from build123d import *

# Parameters (mm, degrees)
SKETCH_1_W      = 60
SKETCH_1_H      = 44
EXTRUDE_3_DEPTH = 2.5
SKETCH_4_R      = 1.5
EXTRUDE_4_DEPTH = 17.5
EXTRUDE_START   = -17.5
SKETCH_5_R      = 1.5
EXTRUDE_5_DEPTH = 17.5


with BuildPart() as part:
    # 草图1 → 凸台-拉伸3 (new body)
    with BuildSketch(Plane.XY):
        Rectangle(SKETCH_1_W, SKETCH_1_H)
    extrude(amount=EXTRUDE_3_DEPTH)

    # 草图4 → 凸台-拉伸4 (add)
    with BuildSketch(Plane(origin=(30, 0, 0), x_dir=(0, 0, -1), z_dir=(1, 0, 0))):
        with BuildLine():
            Line((0, -22), (0, -13))
            Line((0, -13), (4.271805299, -24.258355855))
            ThreePointArc((4.271805299, -24.258355855), (1.630618235, -28.942618859), (-2.500551622, -25.5))
            Line((-2.500551622, -25.5), (-2.500551622, -22))
            Line((-2.500551622, -22), (0, -22))
        make_face()
        with Locations((0.999448378, -25.5)):
            Circle(SKETCH_4_R, mode=Mode.SUBTRACT)
    extrude(amount=-EXTRUDE_4_DEPTH)

    # 草图5 → 凸台-拉伸5 (add)
    with BuildSketch(Plane.ZY.offset(30).offset(EXTRUDE_START)):
        with BuildLine():
            Line((2.5, -22), (0, -22))
            Line((0, -22), (0, -13))
            Line((0, -13), (-4.271805299, -24.258355855))
            ThreePointArc((-4.271805299, -24.258355855), (-1.630618235, -28.942618859), (2.500551622, -25.5))
            Line((2.500551622, -25.5), (2.5, -22))
        make_face()
        with Locations(Location((-0.999448378, -25.5, 0), (0, 0, 180))):
            Circle(SKETCH_5_R, mode=Mode.SUBTRACT)
    extrude(amount=EXTRUDE_5_DEPTH)


solid = part.part
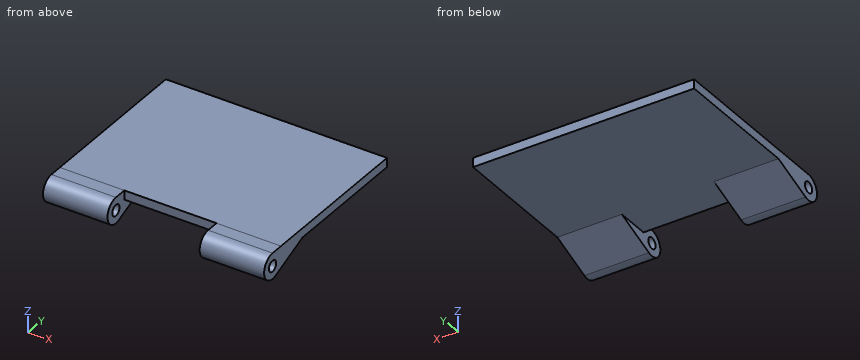
For this review, take the finished solid that the model builds, in its own axes (mm). Round coordinates to 2 decimals unless told otherwise and drop trailing zeros. Write each loop counter-clockwise with the first axis right and the second up, starting at its lowest first coordinate (ties: lowest second). Pieces come first, ordered by that corner, then holes. Notation, with made-up numbers: (30, -31.75) - (75, -31.75) arc R17 cw to (75, -18.75) - close; hole circle Ø11 at (-4.5, -22). An arc over 180 degrees is marked (long way). Use a Markdown table: item, result.
Q1. We need section A-A (x = -18.5). Give the boundary of the cut face in (y, z).
Derived:
| item | result |
|---|---|
| outline | (-25.5, 2.5) arc R3.5 ccw (long way) to (-24.26, -4.27) - (-13, 0) - (22, 0) - (22, 2.5) - (-22, 2.5) - close; hole circle Ø3 at (-25.5, -1) |
Q2. Clearance check with flat-ended pins moving along their axes: pin 1 (0.8 mm diameter, centred on x = -5.5, z = 1, fed in from -Y); pin 2 (4 mm diameter, centred on y = 11, z = -2.5, fed in from -X); pin 3 (22 mm diameter, centred on x = -6, y = 0, fed in from -Z). State where each tip first meets the part, or that it passes through.
Derived:
| item | result |
|---|---|
| pin 1 | stops at y = -22 |
| pin 2 | passes through |
| pin 3 | stops at z = 0 |
Q3. We need section B-B (z = -0.75). Give the boundary of the cut face in (x, y), plus the area to 3 significant figures.
Derived:
| item | result |
|---|---|
| outline | (-30, -28.99) - (-12.5, -28.99) - (-12.5, -26.98) - (-30, -26.98) - close; (-30, -24.02) - (-12.5, -24.02) - (-12.5, -14.98) - (-30, -14.98) - close; (12.5, -28.99) - (30, -28.99) - (30, -26.98) - (12.5, -26.98) - close; (12.5, -24.02) - (30, -24.02) - (30, -14.98) - (12.5, -14.98) - close |
| area | 387 mm2 |
Q4. We need section D-D (y = 16.5). Give the boundary of the cut face in (x, z).
Derived:
| item | result |
|---|---|
| outline | (-30, 0) - (30, 0) - (30, 2.5) - (-30, 2.5) - close |
Q5. Wall thickness on line 1 along Z through (x, y) = (-21, -25.5); line 2 along Z through (x, y) = (6, 0); line 3 along X through (y, z) = (-21.5, -1.75): over which ranges is each line inside the solid? List them lowest first.
Derived:
| item | result |
|---|---|
| line 1 | z = -4.5 to -2.5, 0.5 to 2.5 |
| line 2 | z = 0 to 2.5 |
| line 3 | x = -30 to -12.5, 12.5 to 30 |
